Part model, mm, in its own coordinate system. Round coordinates to 2 decimals unless told otherwise and drop trailing zeros. Order: outer loops, then holes, each group sorted by start corner. A loop starts at its lowest first (then second) coordinate and runs counter-clockwise, first axis right, second up. Notation, with made-up numbers: (6, 74.25) -> (37, 74.25) arc R20 cw to (37, 113.25) -> close; hole circle Ø1 at (10.5, 0). An arc over 180 degrees is marked (long way). Answer as a JSON object with one key per item and string values. Group by question number.
Autodesk Inventor part; units mm, degrees
ref_plane "YZ Plane" through (0, 0, 0) normal (1, 0, 0) x (0, 1, 0)
ref_plane "XZ Plane" through (0, 0, 0) normal (0, 1, 0) x (-1, 0, 0)
ref_plane "XY Plane" through (0, 0, 0) normal (0, 0, 1) x (1, 0, 0)
sketch "Sketch1" plane through (0, 0, 0) normal (0, 0, 1) x (1, 0, 0)
  line L0 (0, 0) -> (224.6, 0)
  line L1 (224.6, 0) -> (224.6, 69.85)
  line L2 (224.6, 69.85) -> (0, 69.85)
  line L3 (0, 69.85) -> (0, 0)
  dimension "d0" = 224.6
  dimension "d1" = 69.85
extrude "Extrusion1" add sketch "Sketch1" along normal blind 2
sketch "Sketch2" plane through (0, 0, 2) normal (0, 0, 1) x (1, 0, 0)
  line L0 (224.6, 0) -> (224.6, 69.85)
  line L1 (224.6, 69.85) -> (0, 69.85)
  line L2 (0, 69.85) -> (0, 0)
  line L3 (0, 0) -> (224.6, 0)
  line L4 (2, 67.85) -> (222.6, 67.85)
  line L5 (222.6, 67.85) -> (222.6, 2)
  line L6 (222.6, 2) -> (2, 2)
  line L7 (2, 2) -> (2, 67.85)
  dimension "d4" = 2
extrude "Extrusion2" add sketch "Sketch2" along normal blind 2 contours L4 L5 L6 L7
sketch "Sketch3" plane through (0, 0, 4) normal (0, 0, 1) x (1, 0, 0)
  line L0 (2, 2) -> (222.6, 2) construction
  line L1 (222.6, 2) -> (222.6, 67.85) construction
  line L2 (222.6, 67.85) -> (2, 67.85) construction
  line L3 (2, 67.85) -> (2, 2) construction
  line L4 (2, 67.85) -> (6, 67.85)
  line L5 (6, 67.85) -> (6, 65.85)
  line L6 (6, 65.85) -> (2, 65.85)
  line L7 (2, 65.85) -> (2, 67.85)
  line L8 (222.6, 67.85) -> (218.6, 67.85)
  line L9 (218.6, 67.85) -> (218.6, 65.85)
  line L10 (218.6, 65.85) -> (222.6, 65.85)
  line L11 (222.6, 65.85) -> (222.6, 67.85)
  point P0 (0, 0)
  dimension "d7" = 4
  dimension "d8" = 2
  dimension "d9" = 4
  dimension "d10" = 2
extrude "Extrusion3" cut sketch "Sketch3" against normal blind 2
sketch "Sketch4" plane through (0, 0, 4) normal (0, 0, 1) x (1, 0, 0)
  line L0 (6, 67.85) -> (6, 65.85) construction
  line L1 (6, 65.85) -> (2, 65.85) construction
  line L2 (2, 65.85) -> (2, 2) construction
  line L3 (2, 2) -> (222.6, 2) construction
  line L4 (222.6, 2) -> (222.6, 65.85) construction
  line L5 (222.6, 65.85) -> (218.6, 65.85) construction
  line L6 (218.6, 65.85) -> (218.6, 67.85) construction
  line L7 (218.6, 67.85) -> (6, 67.85) construction
  line L8 (2, 2) -> (24.75, 2) construction
  line L9 (24.75, 2) -> (24.75, 13.5) construction
  line L10 (24.75, 13.5) -> (2, 13.5) construction
  line L11 (2, 13.5) -> (2, 2) construction
  line L12 (16.2953, 6.5) -> (32.5453, 6.5)
  line L13 (32.5453, 6.5) -> (32.5453, 20.5)
  line L14 (32.5453, 20.5) -> (16.2953, 20.5)
  line L15 (16.2953, 20.5) -> (16.2953, 6.5)
  line L16 (16.2953, 6.5) -> (32.5453, 20.5) construction
  line L17 (32.5453, 6.5) -> (16.2953, 20.5) construction
  point P0 (0, 0)
  point P1 (24.4203, 13.5)
  dimension "d13" = 22.75
  dimension "d14" = 11.5
  dimension "d15" = 16.25
  dimension "d16" = 14
extrude "Extrusion4" cut sketch "Sketch4" against normal up to surface (4 mm away)
sketch "Sketch5" plane through (0, 0, 4) normal (0, 0, 1) x (1, 0, 0)
  line L0 (32.5453, 20.5) -> (32.5453, 6.5) construction
  line L1 (32.5453, 6.5) -> (16.2953, 6.5) construction
  line L2 (16.2953, 6.5) -> (16.2953, 20.5) construction
  line L3 (16.2953, 20.5) -> (32.5453, 20.5) construction
  line L4 (6, 67.85) -> (6, 65.85) construction
  line L5 (6, 65.85) -> (2, 65.85) construction
  line L6 (2, 65.85) -> (2, 2) construction
  line L7 (2, 2) -> (222.6, 2) construction
  line L8 (222.6, 2) -> (222.6, 65.85) construction
  line L9 (222.6, 65.85) -> (218.6, 65.85) construction
  line L10 (218.6, 65.85) -> (218.6, 67.85) construction
  line L11 (218.6, 67.85) -> (6, 67.85) construction
  line L12 (32.5453, 20.5) -> (77.7953, 20.5) construction
  line L13 (64.0453, 9.925) -> (91.5453, 9.925)
  line L14 (91.5453, 9.925) -> (91.5453, 57.925)
  line L15 (91.5453, 57.925) -> (64.0453, 57.925)
  line L16 (64.0453, 57.925) -> (64.0453, 9.925)
  line L17 (64.0453, 9.925) -> (91.5453, 57.925) construction
  line L18 (91.5453, 9.925) -> (64.0453, 57.925) construction
  line L19 (77.7953, 20.5) -> (77.7953, 33.925) construction
  point P0 (0, 0)
  dimension "d19" = 45.25
  dimension "d20" = 27.5
  dimension "d21" = 48
extrude "Extrusion5" cut sketch "Sketch5" against normal up to surface (4 mm away)
sketch "Sketch6" plane through (0, 0, 4) normal (0, 0, 1) x (1, 0, 0)
  line L0 (91.5453, 57.925) -> (91.5453, 9.925) construction
  line L1 (91.5453, 9.925) -> (64.0453, 9.925) construction
  line L2 (64.0453, 9.925) -> (64.0453, 57.925) construction
  line L3 (64.0453, 57.925) -> (91.5453, 57.925) construction
  line L4 (32.5453, 20.5) -> (32.5453, 6.5) construction
  line L5 (32.5453, 6.5) -> (16.2953, 6.5) construction
  line L6 (16.2953, 6.5) -> (16.2953, 20.5) construction
  line L7 (16.2953, 20.5) -> (32.5453, 20.5) construction
  line L8 (6, 67.85) -> (6, 65.85) construction
  line L9 (6, 65.85) -> (2, 65.85) construction
  line L10 (2, 65.85) -> (2, 2) construction
  line L11 (2, 2) -> (222.6, 2) construction
  line L12 (222.6, 2) -> (222.6, 65.85) construction
  line L13 (222.6, 65.85) -> (218.6, 65.85) construction
  line L14 (218.6, 65.85) -> (218.6, 67.85) construction
  line L15 (218.6, 67.85) -> (6, 67.85) construction
  line L16 (0, 0) -> (224.6, 0) construction
  line L17 (64.0453, 0) -> (60.2953, 0) construction
  line L18 (60.2953, 0) -> (60.2953, 57.925) construction
  line L19 (60.2953, 57.925) -> (64.0453, 57.925) construction
  line L20 (64.0453, 57.925) -> (64.0453, 0) construction
  line L21 (91.5453, 57.925) -> (95.2953, 57.925) construction
  line L22 (95.2953, 57.925) -> (95.2953, 0) construction
  line L23 (95.2953, 0) -> (91.5453, 0) construction
  line L24 (91.5453, 0) -> (91.5453, 57.925) construction
  line L25 (60.2953, 57.925) -> (64.0453, 57.925)
  line L26 (64.0453, 57.925) -> (64.0453, 0)
  line L27 (64.0453, 0) -> (60.2953, 0)
  line L28 (60.2953, 0) -> (60.2953, 57.925)
  line L29 (91.5453, 0) -> (95.2953, 0)
  line L30 (95.2953, 0) -> (95.2953, 57.925)
  line L31 (95.2953, 57.925) -> (91.5453, 57.925)
  line L32 (91.5453, 57.925) -> (91.5453, 0)
  line L33 (64.0453, 9.925) -> (64.0453, 57.925)
  dimension "d24" = 3.75
  dimension "d25" = 3.75
extrude "Extrusion6" add sketch "Sketch6" along normal blind 4 and the other way blind 2
sketch "Sketch7" plane through (0, 0, 4) normal (0, 0, 1) x (1, 0, 0)
  line L0 (32.5453, 20.5) -> (32.5453, 6.5) construction
  line L1 (32.5453, 6.5) -> (16.2953, 6.5) construction
  line L2 (16.2953, 6.5) -> (16.2953, 20.5) construction
  line L3 (16.2953, 20.5) -> (32.5453, 20.5) construction
  line L4 (91.5453, 57.925) -> (95.2953, 57.925) construction
  line L5 (95.2953, 57.925) -> (95.2953, 2) construction
  line L6 (95.2953, 2) -> (222.6, 2) construction
  line L7 (222.6, 2) -> (222.6, 65.85) construction
  line L8 (222.6, 65.85) -> (218.6, 65.85) construction
  line L9 (218.6, 65.85) -> (218.6, 67.85) construction
  line L10 (218.6, 67.85) -> (6, 67.85) construction
  line L11 (6, 67.85) -> (6, 65.85) construction
  line L12 (6, 65.85) -> (2, 65.85) construction
  line L13 (2, 65.85) -> (2, 2) construction
  line L14 (2, 2) -> (60.2953, 2) construction
  line L15 (60.2953, 2) -> (60.2953, 57.925) construction
  line L16 (60.2953, 57.925) -> (64.0453, 57.925) construction
  line L17 (64.0453, 57.925) -> (91.5453, 57.925) construction
  line L18 (32.5453, 6.5) -> (32.5453, 20.5)
  line L19 (32.5453, 20.5) -> (16.2953, 20.5)
  arc A0 (32.5453, 20.5) -> (16.2953, 20.5) centre (24.4203, 20.5) ccw
  line L20 (64.0453, 9.925) -> (64.0453, 2)
  line L21 (64.0453, 2) -> (91.5453, 2)
  line L22 (91.5453, 2) -> (91.5453, 9.925)
  line L23 (91.5453, 9.925) -> (64.0453, 9.925)
  point P0 (0, 0)
  dimension "d30" = 8.125
extrude "Extrusion7" cut sketch "Sketch7" against normal up to surface (4 mm away) contours L19 A0
properties part number "back"
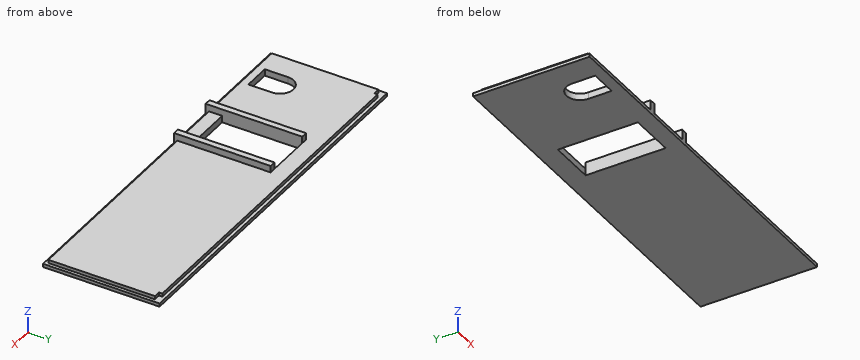
Q1. Band-saw the part on C-C (x = 73). List the corners of the cut face in (y, z) (3 decimals).
Q2. Band-saw the part on B-B (y = 35). List the corners of the cut face in (x, z), plus the area to 3 significant figures.
Q3. Drop flat-ended pins along their axis: pin 1 Ø0.6 at (x, z) = (78, 3.5) entering from -Y; pin 2 Ø1 at (y, z) = (21.5, 3) entering from -X; pin 3 Ø4 at (x, y) = (84.5, 6) entering from +Z. Give the stop position or say it passes through.
Q4. Band-saw the part on A-A (z = 5.25). List the corners of the cut face in (x, y) (3 decimals).
Q5. Wall check: line 1 (X direction, y = 33, z = 2.5); line 2 (X direction, y = 22.5, z = 0.75); line 3 (X direction, y = 29.5, z = 7). Give the ranges that are in metal, low to high. Write a range as [from, to].
Q6. Band-saw the part on D-D (x = 47). List the corners of the cut face in (y, z).
Completed:
{
 "1": {"outline": "(0, 0) -> (9.925, 0) -> (9.925, 4) -> (2, 4) -> (2, 2) -> (0, 2) -> close; (57.925, 0) -> (69.85, 0) -> (69.85, 2) -> (67.85, 2) -> (67.85, 4) -> (57.925, 4) -> close"},
 "2": {"outline": "(0, 0) -> (64.05, 0) -> (64.05, 8) -> (60.3, 8) -> (60.3, 4) -> (2, 4) -> (2, 2) -> (0, 2) -> close; (91.55, 0) -> (224.6, 0) -> (224.6, 2) -> (222.6, 2) -> (222.6, 4) -> (95.3, 4) -> (95.3, 8) -> (91.55, 8) -> close", "area": "810 mm2"},
 "3": {"pin 1": "y = 2", "pin 2": "x = 2", "pin 3": "z = 4"},
 "4": {"outline": "(60.295, 0) -> (64.045, 0) -> (64.045, 57.925) -> (60.295, 57.925) -> close; (91.545, 0) -> (95.295, 0) -> (95.295, 57.925) -> (91.545, 57.925) -> close"},
 "5": {"line 1": "[2, 64.05], [91.55, 222.6]", "line 2": "[0, 16.55], [32.3, 64.05], [91.55, 224.6]", "line 3": "[60.3, 64.05], [91.55, 95.3]"},
 "6": {"outline": "(0, 0) -> (69.85, 0) -> (69.85, 2) -> (67.85, 2) -> (67.85, 4) -> (2, 4) -> (2, 2) -> (0, 2) -> close"}
}
